from build123d import *

# Parameters (mm, degrees)
BOSS_EXTRUDE1_OUTLINE_R = 2
BOSS_EXTRUDE1_DEPTH     = 3
CUT_EXTRUDE2_DEPTH      = 3
CUT_EXTRUDE3_DEPTH      = 58.098511364
FILLET1_R               = 2
FILLET2_R               = 1


# Read off the part's stored shape, not the designer's step: Boss-Extrude1
with BuildPart() as part:
    # Boss-Extrude1 outline → Boss-Extrude1 (new body)
    with BuildSketch(Plane(origin=(0, 0, 0), x_dir=(1, 0, 0), z_dir=(0, 1, 0))):
        with BuildLine():
            ThreePointArc((0, 4.5), (-4.5, 0), (0, -4.5))
            Line((0, -4.5), (51.8, -5))
            ThreePointArc((51.8, -5), (56.8, 0), (51.8, 5))
            Line((51.8, 5), (0, 4.5))
        make_face()
        with Locations((51.8, 0)):
            Circle(BOSS_EXTRUDE1_OUTLINE_R, mode=Mode.SUBTRACT)
    extrude(amount=BOSS_EXTRUDE1_DEPTH)

    # Sketch4 → Cut-Extrude2 (cut)
    with BuildSketch(Plane(origin=(0, 0, 0), x_dir=(-1, 0, 0), z_dir=(0, -1, 0))):
        with BuildLine():
            Line((0, 1.563625245), (0, 0))
            Line((0, 0), (0, -1.436374754))
            ThreePointArc((0, -1.436374754), (1.060634912, -0.997021111), (1.499960925, 0.063625245))
            ThreePointArc((1.499960925, 0.063625245), (1.060634912, 1.124271602), (0, 1.563625245))
        make_face()
        with BuildLine():
            Line((-1.498689077, 0), (0, 0))
            Line((0, 0), (0, 1.563625245))
            ThreePointArc((0, 1.563625245), (-1.082947037, 1.101560863), (-1.498689077, 0))
        make_face()
        with BuildLine():
            Line((0, -1.436374754), (0, 0))
            Line((0, 0), (-1.498689077, 0))
            ThreePointArc((-1.498689077, 0), (-1.037946482, -1.019309755), (0, -1.436374754))
        make_face()
        with BuildLine():
            Line((-1.498689077, 0), (0, 0))
            Line((0, 0), (0, 1.563625245))
            ThreePointArc((0, 1.563625245), (-1.082947037, 1.101560863), (-1.498689077, 0))
        make_face()
    extrude(amount=-CUT_EXTRUDE2_DEPTH, mode=Mode.SUBTRACT)

    # Sketch5 → Cut-Extrude3 (cut, through all)
    with BuildSketch(Plane.XZ):
        with BuildLine():
            Line((51.8, 5), (25.9, 4.75))
            Line((25.9, 4.75), (25.9, 2.25))
            ThreePointArc((25.9, 2.25), (38.916262453, 3.000928167), (51.8, 5))
        make_face()
        with BuildLine():
            Line((25.9, 2.25), (25.9, 4.75))
            Line((25.9, 4.75), (0, 4.5))
            ThreePointArc((0, 4.5), (12.89588572, 2.752084515), (25.9, 2.25))
        make_face()
        with BuildLine():
            Line((51.8, 5), (25.9, 4.75))
            Line((25.9, 4.75), (25.9, 2.25))
            ThreePointArc((25.9, 2.25), (38.916262453, 3.000928167), (51.8, 5))
        make_face()
        with BuildLine():
            Line((25.9, 2.25), (25.9, 4.75))
            Line((25.9, 4.75), (0, 4.5))
            ThreePointArc((0, 4.5), (12.89588572, 2.752084515), (25.9, 2.25))
        make_face()
    extrude(amount=-CUT_EXTRUDE3_DEPTH, mode=Mode.SUBTRACT)

    # Fillet1
    fillet1_edges = [part.edges().sort_by_distance(p)[0] for p in [
        (25.924129047, 3, 2.250230756),
    ]]
    fillet(fillet1_edges, radius=FILLET1_R)

    # Fillet2
    fillet2_edges = [part.edges().sort_by_distance(p)[0] for p in [
        (25.924129047, 0, 2.250230756),
    ]]
    fillet(fillet2_edges, radius=FILLET2_R - 0.0001)  # a hair under: the kernel refuses the full size


solid = part.part
Can you work these out from the model? Positions are in its coordinate system, mm. Give positions to 0.01 mm unless a question says otherwise; leave off trailing zeros. Loops run counter-clockwise (first coordinate to the right, second up) from the corner with the lowest first, then second, coordinate; pieces in that order, holes last. Notation, with made-up numbers: (36.5, -32) -> (74.5, -32) arc R28 ccw to (74.5, 6) -> close; hole circle Ø10 at (79.25, 77.25). An arc over 180 degrees is marked (long way). Write item = value, one per line.
1) Suppose I cut it at C-C on z = -3. Write out the boundary of the cut face in (x, y).
Check result:
outline = (-3.35, 0) -> (55.8, 0) -> (55.8, 3) -> (-3.35, 3) -> close
2) I need wall thicknesses on L1, parallel to X at y = 1.45, z = 0; L2, parallel to Z at x = 51.8, y = 0.85; L3, parallel to X at y = 1.7, z = -0.75. Which ranges of each line are inside material? Lowest first, please. Write a range as from..to.
Check result:
L1 = -4.5..-1.5, 1.5..49.8, 53.8..56.8
L2 = -5..-2, 2..4.99
L3 = -4.44..-1.33, 1.33..49.95, 53.65..56.74
3) Suppose I cut it at B-B on y = 2.2. Write out the boundary of the cut face in (x, z).
Check result:
outline = (-1.24, 4.33) arc R4.5 ccw to (0, -4.5) -> (51.8, -5) arc R5 ccw to (53.02, 4.85) arc R135.83 cw to start; hole circle Ø3 at (0, -0.06); hole circle Ø4 at (51.8, 0)
4) Thinking about a two-plate mould opening in Z: for faces 1 (the cylindrical face through (56.8, 1.5, 0.1)), 2 (the cylindrical face through (53.647, 1.479, 0.766)), 3 (the flat face through (26, 0, -1)), which applies, released by +Z, released by -Z, zero draft, split by the parting line, or undercut?
Check result:
face_1 = split by the parting line
face_2 = undercut
face_3 = zero draft
5) Will these pins go through, and if not, where does the flat tip stop? pin 1 (1 mm diameter, centred on x = 42.5, y = 1, fed in from +Z); pin 2 (5 mm diameter, centred on x = 27.5, z = 4, fed in from -Y).
Check result:
pin_1 = 3.5
pin_2 = 0.03
6) Suppose I cut it at A-A on z = -0.75. Write out the boundary of the cut face in (x, y), then the cut area to 3 significant figures.
Check result:
outline = (-4.44, 0) -> (-1.33, 0) -> (-1.33, 3) -> (-4.44, 3) -> close; (1.33, 0) -> (49.95, 0) -> (49.95, 3) -> (1.33, 3) -> close; (53.65, 0) -> (56.74, 0) -> (56.74, 3) -> (53.65, 3) -> close
area = 164 mm2
